Here's how the part is built. I have some questions about the finished solid (model axes, mm). A direction names the side the tool comes from. Round coordinates to 2 decimals unless told otherwise and drop trailing zeros. Write each loop counter-clockwise with the first axis right and the second up, starting at its lowest first coordinate (ties: lowest second). Pieces come first, ordered by that corner, then holes. Notation, with made-up numbers: (20, 36.25) -> (56, 36.25) arc R16 cw to (56, 54.25) -> close; hole circle Ø3 at (-23.5, -39.5). An arc over 180 degrees is marked (long way). Put each result on its own line as item: value. Start each with the question number.
1. Which directions (+Z, -Z, +X, -X, +Y, -Y) give clear straight access to the entire face, cutting with the end or side of a thin tool? Please do faces 1 (the face through (0, 8, 0)), 2 (the face through (0, -0.95, -31)), 3 (the face through (-18, 6.05, -33)).
2. I need wall thicknesses on probe 1 along X at (y, z) = (7, -28.75); probe 2 along Y at (x, z) = (-18.5, -32.8); probe 3 along X at (y, z) = (8.25, 32). Which ranges of each line are inside material? Lowest first, please. Write a range as from..to.
3. For pin 1 (3 mm diameter, centred on x = 9.5, z = 31.5, fed in from -Y); pin 2 (9 mm diameter, centred on x = -1.5, z = -5.5, fed in from -Y); pin 3 (2 mm diameter, centred on x = 17.5, y = 2.5, fed in from +Z); pin 4 (6 mm diameter, centred on y = 1.5, z = -27, fed in from -X), each with a flat end and sliding along its axis, tell me the tip position at first contact or that it passes through.
4. Suppose I cut it at A-A (z = -28.75). Please give me the cut outline in (x, y).
5. We'd pull the mould along Z, two halves only. Please class faces 4 (the face through (0, -0.95, 19)), 5 (the face through (8.5, 4.9, -30)), 6 (the face through (-16.9, 3.4, -31)): +Z half, -Z half, draft (parallel to the pull), parting line (faces both ways), or undercut.
6. Suppose I cut it at C-C (y = 3.25). Please give me the cut outline in (x, z) (3 decimals).
7. Suppose I cut it at B-B (x = 18.5). Please give me the cut outline in (y, z), then the cut area to 3 significant figures.
8. Suppose I cut it at D-D (x = 6). Please give me the cut outline in (y, z).
```python
from build123d import *

# Parameters (mm, degrees)
BOSS_EXTRUDE2_DEPTH      = 10.5
BOSS_EXTRUDE2_DEPTH_BACK = 0.95
SKETCH3_W                = 30
SKETCH3_H                = 70
SKETCH4_W                = 30
SKETCH4_H                = 35
CUT_EXTRUDE2_DEPTH       = 8.95
SKETCH5_R                = 3.1
CUT_EXTRUDE3_DEPTH       = 48.2784306
SKETCH6_R                = 1.6
CUT_EXTRUDE4_DEPTH       = 40.763079609
SKETCH7_W                = 7
SKETCH7_H                = 7
SKETCH7_R                = 1.6
SKETCH7_R_2              = 1.525130212
BOSS_EXTRUDE3_DEPTH      = 4


with BuildPart() as part:
    # Sketch3 → Boss-Extrude2 (new, two sides: drawn at the far end of the back side and taken through both)
    with BuildSketch(Plane(origin=(0, 0, 0), x_dir=(1, 0, 0), z_dir=(0, 1, 0)).offset(-BOSS_EXTRUDE2_DEPTH_BACK)):
        Rectangle(SKETCH3_W, SKETCH3_H)
    extrude(amount=BOSS_EXTRUDE2_DEPTH + BOSS_EXTRUDE2_DEPTH_BACK)

    # Sketch4 → Cut-Extrude2 (cut)
    with BuildSketch(Plane.XZ.offset(0.95)):
        Rectangle(SKETCH4_W, SKETCH4_H)
    extrude(amount=-CUT_EXTRUDE2_DEPTH, mode=Mode.SUBTRACT)

    # Sketch5 → Cut-Extrude3 (cut, through all)
    with BuildSketch(Plane.ZY.offset(15)):
        with Locations((-23, -1)):
            Circle(SKETCH5_R)
        with Locations((23, -1)):
            Circle(SKETCH5_R)
    extrude(amount=-CUT_EXTRUDE3_DEPTH, mode=Mode.SUBTRACT)

    # Sketch6 → Cut-Extrude4 (cut, through all)
    with BuildSketch(Plane(origin=(0, 10.5, 0), x_dir=(1, 0, 0), z_dir=(0, 1, 0))):
        with Locations(Location((-9.5, 28.75, 0), (0, 0, 270))):
            Circle(SKETCH6_R)
        with Locations(Location((9.5, 28.75, 0), (0, 0, 270))):
            Circle(SKETCH6_R)
        with Locations(Location((-9.5, -31.5, 0), (0, 0, 270))):
            Circle(SKETCH6_R)
        with Locations(Location((9.5, -31.5, 0), (0, 0, 270))):
            Circle(SKETCH6_R)
    extrude(amount=-CUT_EXTRUDE4_DEPTH, mode=Mode.SUBTRACT)

    # Sketch7 → Boss-Extrude3 (add)
    # profile 1 of 2: a face of its own
    with BuildSketch(Plane(origin=(0, 0, -35), x_dir=(-1, 0, 0), z_dir=(0, 0, -1))):
        with Locations((-18.5, 2.55)):
            Rectangle(SKETCH7_W, SKETCH7_H)
        with Locations((-18.5, 2.55)):
            Circle(SKETCH7_R, mode=Mode.SUBTRACT)
    # profile 2 of 2: a face of its own
    with BuildSketch(Plane(origin=(0, 0, -35), x_dir=(-1, 0, 0), z_dir=(0, 0, -1))):
        with Locations((18.5, 2.55)):
            Rectangle(SKETCH7_W, SKETCH7_H)
        with Locations((18.5, 2.55)):
            Circle(SKETCH7_R_2, mode=Mode.SUBTRACT)
    extrude(amount=-BOSS_EXTRUDE3_DEPTH)


solid = part.part
```
Verdict:
1. face 1: +X, -X, -Y
1. face 2: +Z, -Z, +X, -X, -Y
1. face 3: +Z, -Z, -X, +Y
2. probe 1: x = -15..-11.1, -7.9..7.9, 11.1..15
2. probe 2: y = -0.95..1.02, 4.08..6.05
2. probe 3: x = -15..-11.02, -7.98..7.98, 11.02..15
3. pin 1: passes through
3. pin 2: stops at y = 8
3. pin 3: stops at z = -31
3. pin 4: stops at x = -15
4. outline: (-15, -0.95) -> (-11.1, -0.95) -> (-11.1, 10.5) -> (-15, 10.5) -> close; (-7.9, -0.95) -> (7.9, -0.95) -> (7.9, 10.5) -> (-7.9, 10.5) -> close; (11.1, -0.95) -> (15, -0.95) -> (15, 10.5) -> (11.1, 10.5) -> close
5. face 4: draft
5. face 5: undercut
5. face 6: +Z half
6. outline: (-22, -35) -> (-19.855, -35) -> (-19.855, -31) -> (-22, -31) -> close; (-17.145, -35) -> (17.061, -35) -> (17.061, -31) -> (15, -31) -> (15, -17.5) -> (-15, -17.5) -> (-15, -31) -> (-17.145, -31) -> close; (-15, 17.5) -> (15, 17.5) -> (15, 35) -> (-15, 35) -> close; (19.939, -35) -> (22, -35) -> (22, -31) -> (19.939, -31) -> close; hole circle Ø3.2 at (-9.5, -28.75); hole circle Ø3.2 at (-9.5, 31.5); hole circle Ø3.2 at (9.5, -28.75); hole circle Ø3.2 at (9.5, 31.5)
7. outline: (-0.95, -35) -> (0.95, -35) -> (0.95, -31) -> (-0.95, -31) -> close; (4.15, -35) -> (6.05, -35) -> (6.05, -31) -> (4.15, -31) -> close
7. area: 15.2 mm^2
8. outline: (-0.95, -35) -> (10.5, -35) -> (10.5, 35) -> (-0.95, 35) -> (-0.95, 26.1) arc R3.1 cw to (-0.95, 19.9) -> (-0.95, 17.5) -> (8, 17.5) -> (8, -17.5) -> (-0.95, -17.5) -> (-0.95, -19.9) arc R3.1 cw to (-0.95, -26.1) -> close
